The listing builds one solid part. Answer for the finished solid, in the listing's coordinates (mm). Give positions to 0.01 mm unless a question says otherwise; leave off trailing zeros. Write each loop counter-clockwise with the first axis right and the second up, starting at its lowest first coordinate (ties: lowest second). Pieces come first, ordered by that corner, then holes. Notation, with made-up numbers: M 31,14 L 45,14 A5 cw 45,21 Z; hole C -25,-22 d10. An arc over 180 degrees is marked long. Answer as a JSON object with one key per item and string values.
```python
from build123d import *

# Parameters (mm, degrees)
ESQUISSE1_W             = 40
ESQUISSE1_H             = 120
BOSS_EXTRU_1_DEPTH      = 6
ESQUISSE2_W             = 20
ESQUISSE2_H             = 70
ENL_V_MAT_EXTRU_1_DEPTH = 6
ESQUISSE4_R             = 1.5
ENL_V_MAT_EXTRU_2_DEPTH = 6
ESQUISSE5_R             = 3
ENL_V_MAT_EXTRU_3_DEPTH = 3


with BuildPart() as part:
    # Esquisse1 → Boss.-Extru.1 (new body)
    with BuildSketch(Plane.XY):
        with Locations((20, 60)):
            Rectangle(ESQUISSE1_W, ESQUISSE1_H)
    extrude(amount=BOSS_EXTRU_1_DEPTH)

    # Esquisse2 → Enlèv. mat.-Extru.1 (cut)
    with BuildSketch(Plane.XY.offset(6)):
        with Locations((10, 85)):
            Rectangle(ESQUISSE2_W, ESQUISSE2_H)
    extrude(amount=-ENL_V_MAT_EXTRU_1_DEPTH, mode=Mode.SUBTRACT)

    # Esquisse4 → Enlèv. mat.-Extru.2 (cut)
    with BuildSketch(Plane.XY.offset(6)):
        with Locations((3, 47)):
            Circle(ESQUISSE4_R)
        with Locations((37, 3)):
            Circle(ESQUISSE4_R)
        with Locations((30, 50)):
            Circle(ESQUISSE4_R)
    extrude(amount=-ENL_V_MAT_EXTRU_2_DEPTH, mode=Mode.SUBTRACT)

    # Esquisse5 → Enlèv. mat.-Extru.3 (cut)
    with BuildSketch(Plane.XY.offset(6)):
        with Locations((30, 50)):
            Circle(ESQUISSE5_R)
    extrude(amount=-ENL_V_MAT_EXTRU_3_DEPTH, mode=Mode.SUBTRACT)


solid = part.part
```
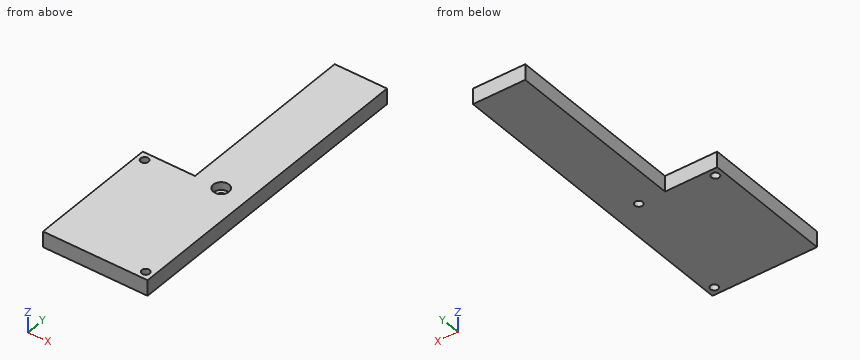
1. A cutting plane is placed at C-C, the plane z = 1.7. Give the vertices of the cut face in (x, y).
Verdict:
{"outline": "M 0,0 L 40,0 L 40,120 L 20,120 L 20,50 L 0,50 Z; hole C 3,47 d3; hole C 30,50 d3; hole C 37,3 d3"}
2. Flat-ended cylindrical pins translate along their axes: pin 1 (4 mm diameter, centred on x = 30, y = 50, fed in from +Z); pin 2 (5 mm diameter, centred on x = 3, y = 47, fed in from +Z); pin 3 (1.8 mm diameter, centred on y = 93.5, z = 3.5, fed in from -X); pin 4 (3 mm diameter, centred on x = 8, z = 2.5, fed in from +Y). Find the tip coordinate at first contact, or state that the pin passes through.
Verdict:
{"pin 1": "stops at z = 3", "pin 2": "stops at z = 6", "pin 3": "stops at x = 20", "pin 4": "stops at y = 50"}
3. A cutting plane is placed at A-A, the plane x = 37. Give the vertices of the cut face in (y, z).
Verdict:
{"outline": "M 0,0 L 1.5,0 L 1.5,6 L 0,6 Z; M 4.5,0 L 120,0 L 120,6 L 4.5,6 Z"}
4. Consider line 1 along Y through (x, z) = (30, 4); line 2 along Y through (x, z) = (7, 4.4); line 3 along X through (y, z) = (74, 3.1). Determine where each line is inside the solid, lowest interval first.
Verdict:
{"line 1": "y = 0 to 47, 53 to 120", "line 2": "y = 0 to 50", "line 3": "x = 20 to 40"}
5. A cutting plane is placed at D-D, the plane x = 30. Give the vertices of the cut face in (y, z).
Verdict:
{"outline": "M 0,0 L 48.5,0 L 48.5,3 L 47,3 L 47,6 L 0,6 Z; M 51.5,0 L 120,0 L 120,6 L 53,6 L 53,3 L 51.5,3 Z"}
6. A cutting plane is placed at B-B, the plane y = 3. Give the vertices of the cut face in (x, z).
Verdict:
{"outline": "M 0,0 L 35.5,0 L 35.5,6 L 0,6 Z; M 38.5,0 L 40,0 L 40,6 L 38.5,6 Z"}
